```python
from build123d import *

# Parameters (mm, degrees)
F1_DEPTH = 100
F2_R     = 6
F3_DEPTH = 200.001
F5_DEPTH = 200.001


with BuildPart() as f1:
    # F0 (on Front) → F1 (new body)
    with BuildSketch(Plane.XZ):
        Polygon((-57.490264, 33.289867), (-63.490264, 33.289867), (-63.490264, -16.710133), (136.509736, -16.710133), (136.509736, 33.289867), (130.509736, 33.289867), (130.509736, -10.710133), (-57.490264, -10.710133), align=None)
    extrude(amount=F1_DEPTH)

    # F2 (on face) → F3 (cut, through all)
    with BuildSketch(Plane.YZ.offset(136.509736)):
        with Locations((-90, 13.289867)):
            Circle(F2_R)
        with Locations((-10, 13.289867)):
            Circle(F2_R)
    extrude(amount=-F3_DEPTH, mode=Mode.SUBTRACT)

    # F4 (on face) → F5 (cut, through all)
    with BuildSketch(Plane.YZ.offset(136.509736)):
        with BuildLine():
            ThreePointArc((-75.70933, 17.848019), (-75.178393, 15.596374), (-75, 13.289867))
            ThreePointArc((-75, 13.289867), (-75.012554, 12.676309), (-75.050194, 12.063778))
            ThreePointArc((-75.050194, 12.063778), (-50, -7.861311), (-24.949806, 12.063778))
            ThreePointArc((-24.949806, 12.063778), (-24.903547, 14.988183), (-24.29067, 17.848019))
            ThreePointArc((-24.29067, 17.848019), (-13.945352, 27.761709), (0, 24.470207))
            Line((0, 24.470207), (0, 33.289867))
            Line((0, 33.289867), (-100, 33.289867))
            Line((-100, 33.289867), (-100, 24.470207))
            ThreePointArc((-100, 24.470207), (-86.054648, 27.761709), (-75.70933, 17.848019))
        make_face()
    extrude(amount=-F5_DEPTH, mode=Mode.SUBTRACT)


solid = f1.part
```
Design review of the part built by this model. Coordinates are the model's own, in mm. A direction names the side the tool comes from. Give positions to 0.01 mm unless a question says otherwise; leave off trailing zeros. Loops run counter-clockwise (first coordinate to the right, second up) from the corner with the lowest first, then second, coordinate; pieces in that order, holes last. Notation, with made-up numbers: (77, 80) -> (107, 80) arc R15 cw to (107, 96) -> close; hole circle Ø4 at (76, 86.25). An arc over 180 degrees is marked (long way). One line per item, written item: value.
Q1. We need section B-B on x = 5. Give the boundary of the cut face in (y, z), and give its area (3 significant figures).
Numbers:
outline: (-100, -16.71) -> (0, -16.71) -> (0, -10.71) -> (-100, -10.71) -> close
area: 600 mm^2
Q2. We need section D-D on y = -86.5. Give the boundary of the cut face in (x, z).
Numbers:
outline: (-63.49, -16.71) -> (136.51, -16.71) -> (136.51, 8.42) -> (130.51, 8.42) -> (130.51, -10.71) -> (-57.49, -10.71) -> (-57.49, 8.42) -> (-63.49, 8.42) -> close; (-63.49, 18.16) -> (-57.49, 18.16) -> (-57.49, 27.88) -> (-63.49, 27.88) -> close; (130.51, 18.16) -> (136.51, 18.16) -> (136.51, 27.88) -> (130.51, 27.88) -> close
Q3. Draft analysis for pull direction X (two halves, no side actions). For faces 1 (the flat face through (-57.49, -49, -9)), 2 (the flat face through (36, -100, -13)), 3 (the flat face through (136.51, -49, -10)), state which applies: pulls with the +X half, pulls with the -X half, needs draft (parallel to the pull), parting line crosses it, or undercut.
Numbers:
face 1: undercut
face 2: needs draft
face 3: pulls with the +X half
Q4. We need section A-A on y = -10. Give the boundary of the cut face in (x, z), and give its area (3 significant figures).
Numbers:
outline: (-63.49, -16.71) -> (136.51, -16.71) -> (136.51, 7.29) -> (130.51, 7.29) -> (130.51, -10.71) -> (-57.49, -10.71) -> (-57.49, 7.29) -> (-63.49, 7.29) -> close; (-63.49, 19.29) -> (-57.49, 19.29) -> (-57.49, 28.29) -> (-63.49, 28.29) -> close; (130.51, 19.29) -> (136.51, 19.29) -> (136.51, 28.29) -> (130.51, 28.29) -> close
area: 1,520 mm^2
Q5. Machinability: for faces 4 (the cylindrical face through (133.552, -24.908, 14.947)), 5 (the cylindrical face through (-60.448, -75.183, 15.628)), 6 (the flat face through (38, -49, -10.71)), 7 (the flat face through (-63.49, -49, -9)), which of the approach directions +Z, -Z, +X, -X, +Y, -Y give a long, thin tool a straight path to every point of the face, cutting with its end or side? Answer none if there is none.
Numbers:
face 4: +X, -X
face 5: +Z, +X, -X
face 6: +Z, +Y, -Y
face 7: +Z, -Z, -X, +Y, -Y
Q6. We need section C-C on y = -29.5. Give the boundary of the cut face in (x, z), and give its area (3 significant figures).
Numbers:
outline: (-63.49, -16.71) -> (136.51, -16.71) -> (136.51, 2.33) -> (130.51, 2.33) -> (130.51, -10.71) -> (-57.49, -10.71) -> (-57.49, 2.33) -> (-63.49, 2.33) -> close
area: 1,360 mm^2
Q7. For L1, parallel to Z at x = 132, y = -90; L2, parallel to X at y = -25.5, z = 8; L3, parallel to Z at x = 1, y = -68.5, list the stretches that pass through material, from the lowest coordinate up.
Numbers:
L1: z = -16.71 to 7.29, 19.29 to 28.29
L2: x = -63.49 to -57.49, 130.51 to 136.51
L3: z = -16.71 to -10.71
Q8. For pin 1 Ø2 at (x, y) = (8, -86) entering from +Z, flat-tipped, find the tip position at first contact; note if it passes through.
Numbers:
pin 1: stops at z = -10.71
